```python
from build123d import *

# Parameters (mm, degrees)
SKETCH4_R           = 2.5
BOSS_EXTRUDE2_DEPTH = 32
BOSS_EXTRUDE3_DEPTH = 28.5
SKETCH1_W           = 12
SKETCH1_H           = 23
BOSS_EXTRUDE4_DEPTH = 22


with BuildPart() as part:
    # Sketch4 → Boss-Extrude2 (new body)
    with BuildSketch(Plane(origin=(0, 0, 0), x_dir=(1, 0, 0), z_dir=(0, 1, 0))):
        with Locations((51.314367453, -99.151596437)):
            Circle(SKETCH4_R)
    extrude(amount=BOSS_EXTRUDE2_DEPTH)

    # Sketch3 → Boss-Extrude3 (add)
    with BuildSketch(Plane(origin=(0, 0, 0), x_dir=(1, 0, 0), z_dir=(0, 1, 0))):
        with BuildLine():
            Line((48.814367453, -106.151596437), (48.814367453, -104.605952495))
            ThreePointArc((48.814367453, -104.605952495), (51.314367453, -93.151596437), (53.814367453, -104.605952495))
            Line((53.814367453, -104.605952495), (53.814367453, -106.151596437))
            ThreePointArc((53.814367453, -106.151596437), (51.314367453, -108.651596437), (48.814367453, -106.151596437))
        make_face()
    extrude(amount=BOSS_EXTRUDE3_DEPTH)

    # Sketch1 → Boss-Extrude4 (add)
    with BuildSketch(Plane(origin=(0, 0, 0), x_dir=(1, 0, 0), z_dir=(0, 1, 0))):
        with Locations((51.314367453, -104.651596437)):
            Rectangle(SKETCH1_W, SKETCH1_H)
    extrude(amount=BOSS_EXTRUDE4_DEPTH)


solid = part.part
```
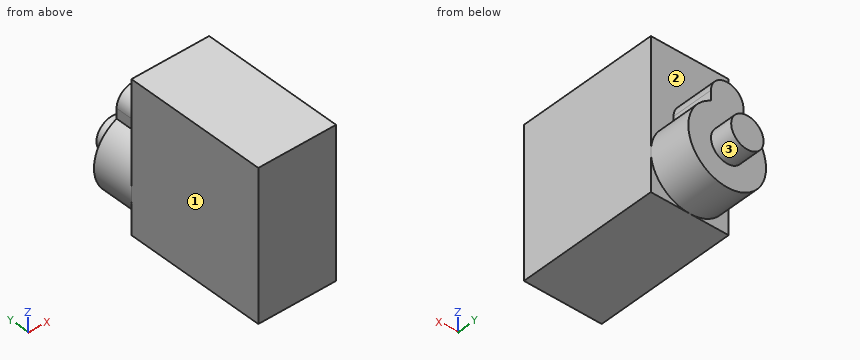
The model under review builds one solid part; all positions refer to its coordinate system, in mm. Face numbers are marked on the shaded views. A direction names the side the tool comes from. Round coordinates to 2 decimals unless told otherwise and drop trailing zeros. Order: outer loops, then holes, each group sorted by start corner. A loop starts at its lowest first (then second) coordinate and runs counter-clockwise, first axis right, second up. Notation, with made-up numbers: (28, 18) - (52, 18) arc R22 cw to (52, 57) - close; hole circle Ø2 at (-30, 57.5). An arc over 180 degrees is marked (long way). Answer in a Markdown table with one row per item.
(1) Take a section at A-A on x = 46.5. Write out the cut boundary in (y, z).
Result set:
| item | result |
|---|---|
| outline | (0, 93.15) - (22, 93.15) - (22, 95.57) - (28.5, 95.57) - (28.5, 102.73) - (22, 102.73) - (22, 116.15) - (0, 116.15) - close |
(2) Clearance check with flat-ended pins moving along their axes: P1, Ø1.2, axis at y = 27, z = 105.5, coming from the +X side; P2, Ø1.8, axis at x = 48.5, z = 97, coming from the +Y side; P3, Ø0.8, axis at y = 24, z = 105.5, coming from the -X side. State where each tip first meets the part, or that it passes through.
Result set:
| item | result |
|---|---|
| P1 | stops at x = 53.81 |
| P2 | stops at y = 28.5 |
| P3 | stops at x = 48.81 |
(3) Take a section at C-C on y = 27. Write out the cut boundary in (x, z), plus the area to 3 significant figures.
Result set:
| item | result |
|---|---|
| outline | (48.81, 104.61) arc R6 ccw (long way) to (53.81, 104.61) - (53.81, 106.15) arc R2.5 ccw to (48.81, 106.15) - close |
| area | 129 mm2 |
(4) Take a section at B-B on z = 109.5. Write out the cut boundary in (x, y), plus the area to 3 significant figures.
Result set:
| item | result |
|---|---|
| outline | (45.31, 0) - (57.31, 0) - (57.31, 22) - (45.31, 22) - close |
| area | 264 mm2 |
(5) Take a section at D-D on x = 54.5. Write out the cut boundary in (y, z), plus the area to 3 significant figures.
Result set:
| item | result |
|---|---|
| outline | (0, 93.15) - (22, 93.15) - (22, 94.07) - (28.5, 94.07) - (28.5, 104.24) - (22, 104.24) - (22, 116.15) - (0, 116.15) - close |
| area | 572 mm2 |
(6) Machinability: for the marked faces 1, 2 and 3, which of the approach directions +Z, -Z, +X, -X, +Y, -Y give a long, thin tool a straight path to every point of the face, cutting with its end or side? Answer none if there is none.
Result set:
| item | result |
|---|---|
| face 1 | +Z, -Z, -X, +Y, -Y |
| face 2 | +Z, +Y |
| face 3 | +Y |
(7) For line 1 (Y direction, x = 55.5, z = 114.25); line 2 (Y direction, x = 47.5, z = 99); line 3 (X direction, y = 27, z = 105.5), list the stretches that pass through material, from the lowest coordinate up. Write a range as from..to.
Result set:
| item | result |
|---|---|
| line 1 | y = 0..22 |
| line 2 | y = 0..28.5 |
| line 3 | x = 48.81..53.81 |
